The listing builds one solid part. Answer for the finished solid, in the listing's coordinates (mm). A direction names the side the tool comes from. Round coordinates to 2 decimals unless told otherwise and drop trailing zeros. Order: outer loops, then holes, each group sorted by start corner. A loop starts at its lowest first (then second) coordinate and runs counter-clockwise, first axis right, second up. Notation, with made-up numbers: (75, 43.5) -> (79, 43.5) arc R17 cw to (79, 60.5) -> close; hole circle Ø10 at (-23.75, 45.25). An arc over 180 degrees is marked (long way). Return JSON: item names as keys, results as strings. Group by question number.
(1) The part is cut by section B-B (x = -4). Determine the outline of the cut face in (y, z).
(2) The part is cut by section D-D (z = 22). Determine the outline of the cut face in (x, y), plus the area to 3 significant figures.
(3) The part is cut by section A-A (y = 8). Determine the outline of the cut face in (x, z).
(4) Determine the mould class of faces 6 (the face through (-1.35, 10.31, 9.17)), 7 (the face through (10.635, 3.349, 1.602)), 8 (the face through (-16.248, 0.11, 21.558)), 9 (the face through (1, -12, 4.75)) for opening direction X: +X half, -X half, draft (parallel to the pull), parting line (faces both ways), or undercut.
(5) Consider line 1 (Z direction, x = 12.5, y = 6); line 2 (Y direction, x = 0, z = 5.5); line 3 (Y direction, x = 0, z = 4.5). Determine where each line is inside the solid, lowest interval first. Write a range as [from, to].
(6) Which of the six approach directions +Z, -Z, +X, -X, +Y, -Y give full straight-line access (tool end or side, diameter ignored) to faces 1 (the face through (-12.46, 1.27, 9.8)), 2 (the face through (11.252, 0.11, 21.558)), 3 (the face through (4, -11, 15.1)), 4 (the face through (12.51, 1.23, 9.8)), 5 (the face through (-11, -4, 3.25))?
(7) Each of these flat-tipped pins is pushed along its axis until it touches: pin 1 (6 mm diameter, centred on y = -11, z = 3.5, fed in from +X); pin 2 (1 mm diameter, centred on x = -9.5, y = 5, fed in from +Z); pin 3 (1 mm diameter, centred on y = -10, z = 13, fed in from -X); pin 4 (8.5 mm diameter, centred on x = 0.5, y = 4.5, fed in from -Z). Where does it stop, or does it pass through?
(8) The part is cut by section C-C (z = 9). Determine the outline of the cut face in (x, y).
from build123d import *

# Parameters (mm, degrees)
F0_R     = 11.15
F0_R_2   = 10.4
F1_DEPTH = 18.6
F2_START = 3.25
F0_R_3   = 14.1
F2_DEPTH = 1.5
F3_R     = 17.2
F3_R_2   = 11.15
F3_R_3   = 10.4
F4_DEPTH = 3.5
F5_R     = 2.5
F6_DEPTH = 7
F7_SIZE  = 1
F9_DEPTH = 10.25


with BuildPart() as f1:
    # F0 (on Top) → F1 (new body)
    with BuildSketch(Plane.XY):
        Circle(F0_R)
        Circle(F0_R_2, mode=Mode.SUBTRACT)
    extrude(amount=F1_DEPTH)

    # F0 (on Top) → F2 (join)
    with BuildSketch(Plane.XY.offset(F2_START)):
        Circle(F0_R_3)
        Circle(F0_R, mode=Mode.SUBTRACT)
    extrude(amount=F2_DEPTH)

    # F3 (on face) → F4 (join)
    with BuildSketch(Plane.XY.offset(18.6)):
        Circle(F3_R)
        Circle(F3_R_2, mode=Mode.SUBTRACT)
        Circle(F3_R_2)
        Circle(F3_R_3, mode=Mode.SUBTRACT)
    extrude(amount=-F4_DEPTH)

    # F5 (on face) → F6 (join)
    with BuildSketch(Plane.XY.offset(18.6)):
        with Locations((13.75, 0)):
            Circle(F5_R)
        with Locations((-13.75, 0)):
            Circle(F5_R)
    extrude(amount=F6_DEPTH)

    # F7
    f7_edges = [f1.edges().sort_by_distance(p)[0] for p in [
        (-16.25, 0, 25.6),
        (11.25, 0, 25.6),
    ]]
    chamfer(f7_edges, length=F7_SIZE)

    # F8 (on face) → F9 (join)
    with BuildSketch(Plane.XY.offset(4.75)):
        with BuildLine():
            Line((10.8661170618, -2.5), (14.1, 0))
            Line((14.1, 0), (10.8661170618, 2.5))
            ThreePointArc((10.8661170618, 2.5), (11.0788019487, 1.2580331397), (11.15, 0))
            ThreePointArc((11.15, 0), (11.0788019487, -1.2580331397), (10.8661170618, -2.5))
        make_face()
        with BuildLine():
            Line((-10.8661170618, 2.5), (-14.1, 0))
            Line((-14.1, 0), (-10.8661170618, -2.5))
            ThreePointArc((-10.8661170618, -2.5), (-11.15, 0), (-10.8661170618, 2.5))
        make_face()
    extrude(amount=F9_DEPTH)


solid = f1.part
Answer below:
{
 "1": {"outline": "(-16.73, 15.1) -> (-10.41, 15.1) -> (-10.41, 4.75) -> (-13.52, 4.75) -> (-13.52, 3.25) -> (-10.41, 3.25) -> (-10.41, 0) -> (-9.6, 0) -> (-9.6, 18.6) -> (-16.73, 18.6) -> close; (9.6, 0) -> (10.41, 0) -> (10.41, 3.25) -> (13.52, 3.25) -> (13.52, 4.75) -> (10.41, 4.75) -> (10.41, 15.1) -> (16.73, 15.1) -> (16.73, 18.6) -> (9.6, 18.6) -> close"},
 "2": {"outline": "circle Ø5 at (-13.75, 0); circle Ø5 at (13.75, 0)", "area": "39.3 mm²"},
 "3": {"outline": "(-15.23, 15.1) -> (-7.77, 15.1) -> (-7.77, 4.75) -> (-11.61, 4.75) -> (-11.61, 3.25) -> (-7.77, 3.25) -> (-7.77, 0) -> (-6.65, 0) -> (-6.65, 18.6) -> (-15.23, 18.6) -> close; (6.65, 0) -> (7.77, 0) -> (7.77, 3.25) -> (11.61, 3.25) -> (11.61, 4.75) -> (7.77, 4.75) -> (7.77, 15.1) -> (15.23, 15.1) -> (15.23, 18.6) -> (6.65, 18.6) -> close"},
 "4": {"face 6": "undercut", "face 7": "parting line", "face 8": "undercut", "face 9": "draft"},
 "5": {"line 1": "z = [3.25, 4.75], [15.1, 18.6]", "line 2": "y = [-11.15, -10.4], [10.4, 11.15]", "line 3": "y = [-14.1, -10.4], [10.4, 14.1]"},
 "6": {"face 1": "-X, +Y", "face 2": "+Z", "face 3": "none", "face 4": "+X, +Y", "face 5": "-Z"},
 "7": {"pin 1": "stops at x = 11.61", "pin 2": "stops at z = 18.6", "pin 3": "stops at x = -5.84", "pin 4": "passes through"},
 "8": {"outline": "(-14.1, 0) -> (-10.87, -2.5) arc R11.15 ccw to (10.87, -2.5) -> (14.1, 0) -> (10.87, 2.5) arc R11.15 ccw to (-10.87, 2.5) -> close; hole circle Ø20.8 at (0, 0)"}
}
